Read the model definition and answer for the solid it produces. Units are mm, in the model's axes. Face numbers are marked on the shaded views. A direction names the side the tool comes from. Coordinates: 2 decimals unless noted, no trailing zeros. Order: outer loops, then holes, each group sorted by start corner. A loop starts at its lowest first (then second) coordinate and runs counter-clockwise, first axis right, second up. Notation, with made-up numbers: (-4, 28.25) -> (33, 28.25) arc R26 cw to (33, 45.25) -> close; hole circle Ø6 at (-29.75, 20.25). An arc over 180 degrees is marked (long way). Use CSV: the item, a comma, the result in double quotes.
```python
from build123d import *

# Parameters (mm, degrees)
SKETCH1_W           = 100
SKETCH1_H           = 25
BOSS_EXTRUDE1_DEPTH = 3
SKETCH2_W           = 30
SKETCH2_H           = 25
BOSS_EXTRUDE2_DEPTH = 5
SKETCH5_R           = 1.6
CUT_EXTRUDE2_DEPTH  = 53.156015952
SKETCH6_W           = 26
SKETCH6_H           = 6
CUT_EXTRUDE3_DEPTH  = 57.124860802
FILLET1_R           = 7.5
SKETCH7_R           = 1.5
BOSS_EXTRUDE3_DEPTH = 4
BOSS_EXTRUDE4_START = 5
SKETCH9_W           = 30
SKETCH9_H           = 25
SKETCH9_R           = 1.6
BOSS_EXTRUDE4_DEPTH = 5


with BuildPart() as part:
    # Sketch1 → Boss-Extrude1 (new body)
    with BuildSketch(Plane(origin=(0, 0, 0), x_dir=(1, 0, 0), z_dir=(0, 1, 0))):
        Rectangle(SKETCH1_W, SKETCH1_H)
    extrude(amount=BOSS_EXTRUDE1_DEPTH)

    # Sketch2 → Boss-Extrude2 (add)
    with BuildSketch(Plane.XZ):
        Rectangle(SKETCH2_W, SKETCH2_H)
    extrude(amount=BOSS_EXTRUDE2_DEPTH)

    # Sketch5 → Cut-Extrude2 (cut, through all)
    with BuildSketch(Plane.XZ.offset(5)):
        with Locations(Location((8, 0, 0), (0, 0, 270))):
            Circle(SKETCH5_R)
        with Locations(Location((0, -8, 0), (0, 0, 270))):
            Circle(SKETCH5_R)
        with Locations(Location((-8, 0, 0), (0, 0, 270))):
            Circle(SKETCH5_R)
        with Locations(Location((0, 8, 0), (0, 0, 270))):
            Circle(SKETCH5_R)
    extrude(amount=-CUT_EXTRUDE2_DEPTH, mode=Mode.SUBTRACT)

    # Sketch6 → Cut-Extrude3 (cut, through all)
    with BuildSketch(Plane(origin=(0, 0, -12.5), x_dir=(-1, 0, 0), z_dir=(0, 0, -1))):
        Rectangle(SKETCH6_W, SKETCH6_H)
    extrude(amount=-CUT_EXTRUDE3_DEPTH, mode=Mode.SUBTRACT)

    # Fillet1
    # the kernel refuses this fillet: 7.5 mm, written as the material it adds along each edge
    with BuildSketch(Plane(origin=(-15, 0, -12.5), x_dir=(-1, 0, 0), z_dir=(0, 0, 1))) as fillet1_piece_1:
        with BuildLine():
            CenterArc((7.071067812, 7.5), FILLET1_R, 199.471220634, 70.528779366)
            Line((0, 5), (-0.141421356, 4.95))
            ThreePointArc((-0.141421356, 4.95), (-0.15, 2.5), (-0.15, 0))
            Line((-0.15, 0), (0, -0.15))
            Line((0, -0.15), (7.071067812, -0.15))
            Line((7.071067812, -0.15), (7.071067812, 0))
        make_face()
    extrude(amount=25)
    with BuildSketch(Plane(origin=(15, 0, 12.5), x_dir=(0, -1, 0), z_dir=(0, 0, -1))) as fillet1_piece_2:
        with BuildLine():
            CenterArc((7.5, -7.071067812), FILLET1_R, 109.471220634, 70.528779366)
            Line((0, -7.071067812), (-0.15, -7.071067812))
            Line((-0.15, -7.071067812), (-0.15, 0))
            Line((-0.15, 0), (0, 0.15))
            ThreePointArc((0, 0.15), (2.5, 0.15), (4.95, 0.141421356))
            Line((4.95, 0.141421356), (5, 0))
        make_face()
    extrude(amount=25)
    # the kernel refuses this fillet: 7.5 mm, written as the material it takes off along each edge
    with BuildSketch(Plane(origin=(-13, 3, -30.871173071), x_dir=(-1.5711876244490177e-12, -1.0, 0), z_dir=(0, 0, 1))) as fillet1_2_piece_1:
        with BuildLine():
            CenterArc((7.5, -7.348469228), FILLET1_R, 101.536959033, 78.463040967)
            Line((0, -7.348469228), (-0.15, -7.348469228))
            Line((-0.15, -7.348469228), (-0.15, 0))
            Line((-0.15, 0), (0, 0.15))
            ThreePointArc((0, 0.15), (3, 0.15), (5.97, 0.146969385))
            Line((5.97, 0.146969385), (6, 0))
        make_face()
    extrude(amount=61.742346142, mode=Mode.SUBTRACT)
    with BuildSketch(Plane(origin=(13, 3, -30.871173071), x_dir=(1, 0, 0), z_dir=(0, 0, 1))) as fillet1_2_piece_2:
        with BuildLine():
            CenterArc((7.348469228, -7.5), FILLET1_R, 90, 78.463040967)
            Line((0, -6), (-0.146969385, -5.97))
            ThreePointArc((-0.146969385, -5.97), (-0.15, -3), (-0.15, 0))
            Line((-0.15, 0), (0, 0.15))
            Line((0, 0.15), (7.348469228, 0.15))
            Line((7.348469228, 0.15), (7.348469228, 0))
        make_face()
    extrude(amount=61.742346142, mode=Mode.SUBTRACT)

    # Sketch7 → Boss-Extrude3 (add)
    with BuildSketch(Plane(origin=(0, 3, 0), x_dir=(1, 0, 0), z_dir=(0, 1, 0))):
        with Locations(Location((-40, 0, 0), (0, 0, 270))):
            Circle(SKETCH7_R)
        with Locations(Location((40, 0, 0), (0, 0, 270))):
            Circle(SKETCH7_R)
    extrude(amount=BOSS_EXTRUDE3_DEPTH)

    # Sketch9 → Boss-Extrude4 (add)
    with BuildSketch(Plane.XZ.offset(5).offset(BOSS_EXTRUDE4_START)):
        Rectangle(SKETCH9_W, SKETCH9_H)
        with Locations(Location((0, -8, 0), (0, 0, 270))):
            Circle(SKETCH9_R, mode=Mode.SUBTRACT)
        with Locations(Location((-8, 0, 0), (0, 0, 270))):
            Circle(SKETCH9_R, mode=Mode.SUBTRACT)
        with Locations(Location((8, 0, 0), (0, 0, 270))):
            Circle(SKETCH9_R, mode=Mode.SUBTRACT)
        with Locations(Location((0, 8, 0), (0, 0, 270))):
            Circle(SKETCH9_R, mode=Mode.SUBTRACT)
    extrude(amount=-BOSS_EXTRUDE4_DEPTH)


solid = part.part
```
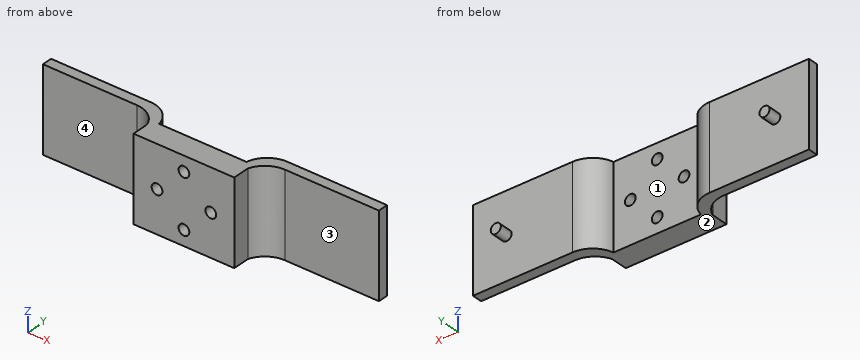
Item 1: Find section A-A, the plane x = -8. Give the vertices of the cut face in (y, z), then the cut area to 3 significant figures.
Return value:
outline,"(-10, -12.5) -> (-3, -12.5) -> (-3, -1.6) -> (-10, -1.6) -> close; (-10, 1.6) -> (-3, 1.6) -> (-3, 12.5) -> (-10, 12.5) -> close"
area,"153 mm^2"
Item 2: Find section C-C, the plane z = -8. Give the vertices of the cut face in (x, y), then the cut area to 3 significant figures.
Return value:
outline,"(-50, 0) -> (-22.07, 0) arc R7.5 cw to (-15, -5) -> (-15, -10) -> (-1.6, -10) -> (-1.6, -3) -> (-13, -3) arc R7.5 ccw to (-20.35, 3) -> (-50, 3) -> close; (1.6, -10) -> (15, -10) -> (15, -5) arc R7.5 cw to (22.07, 0) -> (50, 0) -> (50, 3) -> (20.35, 3) arc R7.5 ccw to (13, -3) -> (1.6, -3) -> close"
area,"419 mm^2"
Item 3: Each of these flat-tipped pins is pushed along its axis until it touches: P1, Ø3.5, axis at x = 0, z = 8, coming from the +Y side; P2, Ø4, axis at x = -8, z = 0, coming from the -Y side; P3, Ø1.5, axis at y = -7.5, z = 6, coming from the -X side; P4, Ø12.5, axis at x = -30.5, z = 3.5, coming from the -Y side. Where does it stop, or does it pass through?
Return value:
P1,"stops at y = -3"
P2,"stops at y = -10"
P3,"stops at x = -15"
P4,"stops at y = 0"
Item 4: A tool of negligible diameter and unlimited length cuts with its end or side. For the marked faces 1, 2, 3 and 4, from which of +Z, -Z, +X, -X, +Y, -Y can it reach the whole face along a straight path? Write none if from no direction.
Return value:
face 1,"+Z, -Z, +Y"
face 2,"-Z, +X, -X, +Y, -Y"
face 3,"+Z, -Z, +X, -Y"
face 4,"+Z, -Z, -X, -Y"
Item 5: Find section D-D, the plane y = -2. Give the vertices of the cut face in (x, z).
Return value:
outline,"(-16.97, -12.5) -> (-13.28, -12.5) -> (-13.28, 12.5) -> (-16.97, 12.5) -> close; (13.28, -12.5) -> (16.97, -12.5) -> (16.97, 12.5) -> (13.28, 12.5) -> close"
Item 6: Find section B-B, the plane y = -7.75. Give the vertices of the cut face in (x, z).
Return value:
outline,"(-15, -12.5) -> (15, -12.5) -> (15, 12.5) -> (-15, 12.5) -> close; hole circle Ø3.2 at (-8, 0); hole circle Ø3.2 at (0, -8); hole circle Ø3.2 at (0, 8); hole circle Ø3.2 at (8, 0)"
Item 7: Straight lines are drawn through the part: line 1 along X through (y, z) = (-7.5, 0); line 2 along X through (y, z) = (0.75, -5.25); line 3 along X through (y, z) = (-6.25, 8). For each, find the intervals that lie inside material, in ascending order.
Return value:
line 1,"x = -15 to -9.6, -6.4 to 6.4, 9.6 to 15"
line 2,"x = -50 to -14.99, 14.99 to 50"
line 3,"x = -15 to -1.6, 1.6 to 15"
